Input: part model. Units: mm. Frame: model coordinates. A direction names the side the tool comes from. Round coordinates to 2 decimals unless told otherwise and drop trailing zeros. Loops run counter-clockwise (first coordinate to the right, second up) from the corner with the lowest first, then second, coordinate; pieces in that order, holes last. Notation, with made-up numbers: (-15, -2) -> (38, -2) arc R32 cw to (38, 25) -> close; hole circle Ø5 at (-12, 55). An arc over 180 degrees is marked (long way). Answer in a Markdown table with one row per item. Add a question column.
Q1. Section C-C, the plane z = -14.75. Output: boundary loops of the cut face in (x, y).
Q2. Mould query, pull axis Y, two halves, no side actions, for faces 1 (the face through (-0.688, -3.242, -16.593)), 2 (the face through (-7.9, -8.4, 0)), 3 (the face through (-5, -1.588, -8)). Classes: pulls with the +Y half, pulls with the -Y half, needs draft (parallel to the pull), parting line crosses it, or undercut.
Q3. Section B-B, the plane x = 0. Output: boundary loops of the cut face in (y, z), and give its area (3 significant figures).
Q4. Section A-A, the plane y = -6.35. Give the number of separate pieces and of enclosed holes in the cut face, and give its area (3 significant figures).
Q5. Reachability of faces 4 (the face through (-6.35, -5, -13)), 5 (the face through (0, -5, -7.144)), 6 (the face through (6.35, -5, -14)), 7 (the face through (0, -5, -19.844)) from +Z, -Z, +X, -X, +Y, -Y: full face, straight path, thin tool, end or side. Return the list, or none.
Q6. Pin query (flat end, axial travel): pin 1 (6 mm diameter, centred on y = -6, z = -14.5, fed in from +X); pin 2 (4.5 mm diameter, centred on x = 6.35, y = -6.35, fed in from -Z); pin 3 (5 mm diameter, centred on x = -5, z = -22, fed in from -Y). Return the tip coordinate at first contact, or that it passes through.
Q7. Ray query, L1, parallel to X at y = -6.35, z = 0.2; L2, parallel to Z at x = 0, y = -2.25; L3, parallel to Z at x = 0, y = -0.25. Return the intervals inside material, ascending. Write a range as from..to.
Q8. Section D-D, the plane y = -19.05. Output: boundary loops of the cut face in (x, z), and give its area (3 significant figures).
```python
from build123d import *

# Parameters (mm, degrees)
ESQUISSE2_W             = 25.4
ESQUISSE2_H             = 3.175
BOSS_EXTRU_1_DEPTH      = 6.35
ESQUISSE5_R             = 3.175
ENL_V_MAT_EXTRU_1_DEPTH = 34.3375
ESQUISSE7_R             = 2.569510145
ENL_V_MAT_EXTRU_2_DEPTH = 38.060560658


with BuildPart() as part:
    # Balayage1: sweep along a path in Esquisse1
    with BuildLine(Plane(origin=(0, 0, 0), x_dir=(0, 0, -1), z_dir=(1, 0, 0))) as balayage1_path:
        Line((25.4, 0), (0, 0))
        Line((0, 0), (0, -25.4))
    # Esquisse2 → Balayage1 (sweep)
    with BuildSketch(Plane(origin=(0, -25.4, 0), x_dir=(-1, 0, 0), z_dir=(0, 1, 0))):
        Rectangle(ESQUISSE2_W, ESQUISSE2_H)
    sweep(path=balayage1_path.line, transition=Transition.RIGHT)

    # Esquisse3 → Boss.-Extru.1 (add)
    with BuildSketch(Plane.XZ.offset(1.5875)):
        Polygon((2.630256121, -19.84375), (6.35, -16.124006121), (6.35, -10.863493879), (2.630256121, -7.14375), (-2.630256121, -7.14375), (-6.35, -10.863493879), (-6.35, -16.124006121), (-2.630256121, -19.84375), align=None)
    extrude(amount=BOSS_EXTRU_1_DEPTH)

    # Esquisse5 → Enlèv. mat.-Extru.1 (cut, through all)
    with BuildSketch(Plane.XZ.offset(7.9375)):
        with Locations((0, -13.49375)):
            Circle(ESQUISSE5_R)
    extrude(amount=-ENL_V_MAT_EXTRU_1_DEPTH, mode=Mode.SUBTRACT)

    # Esquisse7 → Enlèv. mat.-Extru.2 (cut, through all)
    with BuildSketch(Plane(origin=(0, 0, -1.5875), x_dir=(-1, 0, 0), z_dir=(0, 0, -1))):
        with Locations(Location((-6.35, -19.05, 0), (0, 0, 90))):
            Circle(ESQUISSE7_R)
        with Locations(Location((-6.35, -6.35, 0), (0, 0, 90))):
            Circle(ESQUISSE7_R)
        with Locations(Location((6.35, -19.05, 0), (0, 0, 90))):
            Circle(ESQUISSE7_R)
        with Locations(Location((6.35, -6.35, 0), (0, 0, 90))):
            Circle(ESQUISSE7_R)
    extrude(amount=-ENL_V_MAT_EXTRU_2_DEPTH, mode=Mode.SUBTRACT)


solid = part.part
```
Answer block:
| question | item | result |
|---|---|---|
| 1 | outline | (-12.7, -1.59) -> (-6.35, -1.59) -> (-6.35, -7.94) -> (-2.92, -7.94) -> (-2.92, 1.59) -> (-12.7, 1.59) -> close; (2.92, -7.94) -> (6.35, -7.94) -> (6.35, -1.59) -> (12.7, -1.59) -> (12.7, 1.59) -> (2.92, 1.59) -> close |
| 2 | face 1 | needs draft |
| 2 | face 2 | undercut |
| 2 | face 3 | pulls with the -Y half |
| 3 | outline | (-25.4, -1.59) -> (-1.59, -1.59) -> (-1.59, -7.14) -> (-7.94, -7.14) -> (-7.94, -10.32) -> (1.59, -10.32) -> (1.59, 1.59) -> (-25.4, 1.59) -> close; (-7.94, -19.84) -> (-1.59, -19.84) -> (-1.59, -25.4) -> (1.59, -25.4) -> (1.59, -16.67) -> (-7.94, -16.67) -> close |
| 3 | area | 181 mm^2 |
| 4 | separate pieces | 4 |
| 4 | enclosed holes | 1 |
| 4 | area | 150 mm^2 |
| 5 | face 4 | -Z, -X, -Y |
| 5 | face 5 | +X, -X, -Y |
| 5 | face 6 | -Z, +X, -Y |
| 5 | face 7 | -Z, +X, -X, -Y |
| 6 | pin 1 | x = 6.35 |
| 6 | pin 2 | z = -18.37 |
| 6 | pin 3 | y = -1.59 |
| 7 | L1 | -12.7..-8.92, -3.78..3.78, 8.92..12.7 |
| 7 | L2 | -19.84..-16.67, -10.32..-7.14, -1.59..1.59 |
| 7 | L3 | -25.4..-16.67, -10.32..1.59 |
| 8 | outline | (-12.7, -1.59) -> (-8.92, -1.59) -> (-8.92, 1.59) -> (-12.7, 1.59) -> close; (-3.78, -1.59) -> (3.78, -1.59) -> (3.78, 1.59) -> (-3.78, 1.59) -> close; (8.92, -1.59) -> (12.7, -1.59) -> (12.7, 1.59) -> (8.92, 1.59) -> close |
| 8 | area | 48.0 mm^2 |
